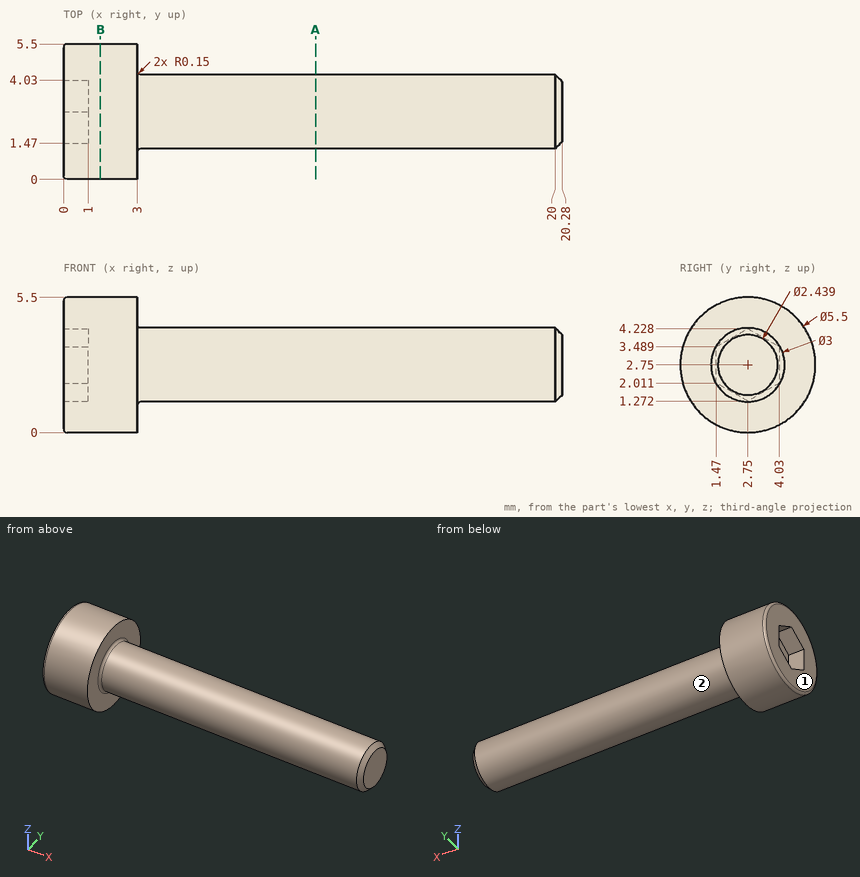
The drawing under review shows one solid part. Ordinate dimensions are in mm from its lowest x, y, z. A direction names the side the tool comes from. Round coordinates to 2 decimals unless told otherwise and drop trailing zeros. Order: outer loops, then holes, each group sorted by start corner. A loop starts at its lowest first (then second) coordinate and runs counter-clockwise, first axis right, second up. Notation, with made-up numbers: M -34.75,1 L -21.75,1 A18 ccw -21.75,26 Z; hole C 89.5,-8 d4. An arc over 180 degrees is marked long. Answer as CSV lines item,"result". Start each with the question number.
1) Tool access review of the marked faces 1 and 2: name each direction out of +Z, -Z, +X, -X, +Y, -Y from which nothing blocks a thin tool from reaching the whole face with its end or side.
2) Add section A-A (x = 10.25). Give the boundary of the cut face in (y, z).
3) Add section B-B (x = 1.5). Give the boundary of the cut face in (y, z).
4) For pin 1 Ø1 at (x, y) = (12.5, 1) entering from +Z; pin 2 Ø2 at (x, z) = (17, 2) entering from -Y; pin 3 Ø3 at (y, z) = (4.5, 0.5) entering from +X, all flat-tipped, find the tip position at first contact; note any pin that passes through.
5) Wall thickness on line 1 along X through (y, z) = (3.35, 5.3); line 2 along X through (y, z) = (3.2, 3.15); line 3 along Y through (x, z) = (12.25, 2.65): over which ranges is each line inside the solid? List them lowest first. Write a range as [from, to].
Resolved:
1,face 1,"+Z, -Z, -X, +Y, -Y"
1,face 2,"+X"
2,outline,"C 2.75,2.75 d3"
3,outline,"C 2.75,2.75 d5.5"
4,pin 1,"z = 3.58"
4,pin 2,"y = 1.25"
4,pin 3,"x = 20.15"
5,line 1,"[0, 3]"
5,line 2,"[1, 20.28]"
5,line 3,"[1.25, 4.25]"
